The figure shows three views and two pictorial views of one solid part (mm, origin at its lowest corner). Answer the questions. A direction names the side the tool comes from. Give positions to 0.01 mm unless a question says otherwise; leave off trailing zeros. Write each loop counter-clockwise with the first axis right and the second up, starting at its lowest first coordinate (ties: lowest second). Pieces come first, ordered by that corner, then holes. Notation, with made-up numbers: (71, 11) - (106, 11) arc R27 cw to (106, 28) - close; hole circle Ø11 at (-2, 23.5). An arc over 180 degrees is marked (long way). Answer as CSV lines item,"result". Start each with the question number.
(1) Find section B-B (y = 42). Write down the section's boundary in (x, z).
(2) For the marked faces 1 and 2, determine the directions among +Z, -Z, +X, -X, +Y, -Y from which every point of the face is accessible in a straight line to the end or side of a thin tool.
(3) Straight lines are drawn through the part: probe 1 along Y at (x, z) = (13.5, 29.5); probe 2 along Y at (x, z) = (24.35, 25.4) (1 decimal); probe 3 along X at (y, z) = (46.5, 35). For each, find the intervals that lie inside material, in ascending order.
(4) For a pull along X with two mould halves and no side action, classify the marked faces 3, 4, 5 and 6 as pulls with the +X half, pulls with the -X half, needs draft (parallel to the pull), parting line crosses it, or undercut.
(5) Find section C-C (z = 25.4). Write down the section's boundary in (x, y) (1 decimal), then the cut area to 3 significant figures.
(6) Find section A-A (x = 7). Write down the section's boundary in (y, z), then the cut area to 3 significant figures.
(7) Find section D-D (z = 46.5). Write down the section's boundary in (x, y).
(8) Each of these flat-tipped pins is pushed along its axis until it touches: pin 1 Ø4 at (y, z) = (37, 20) entering from +X; pin 2 Ø3.5 at (x, z) = (13.51, 12.7) entering from +Y (3 decimals). Where does it stop, or does it pass through?
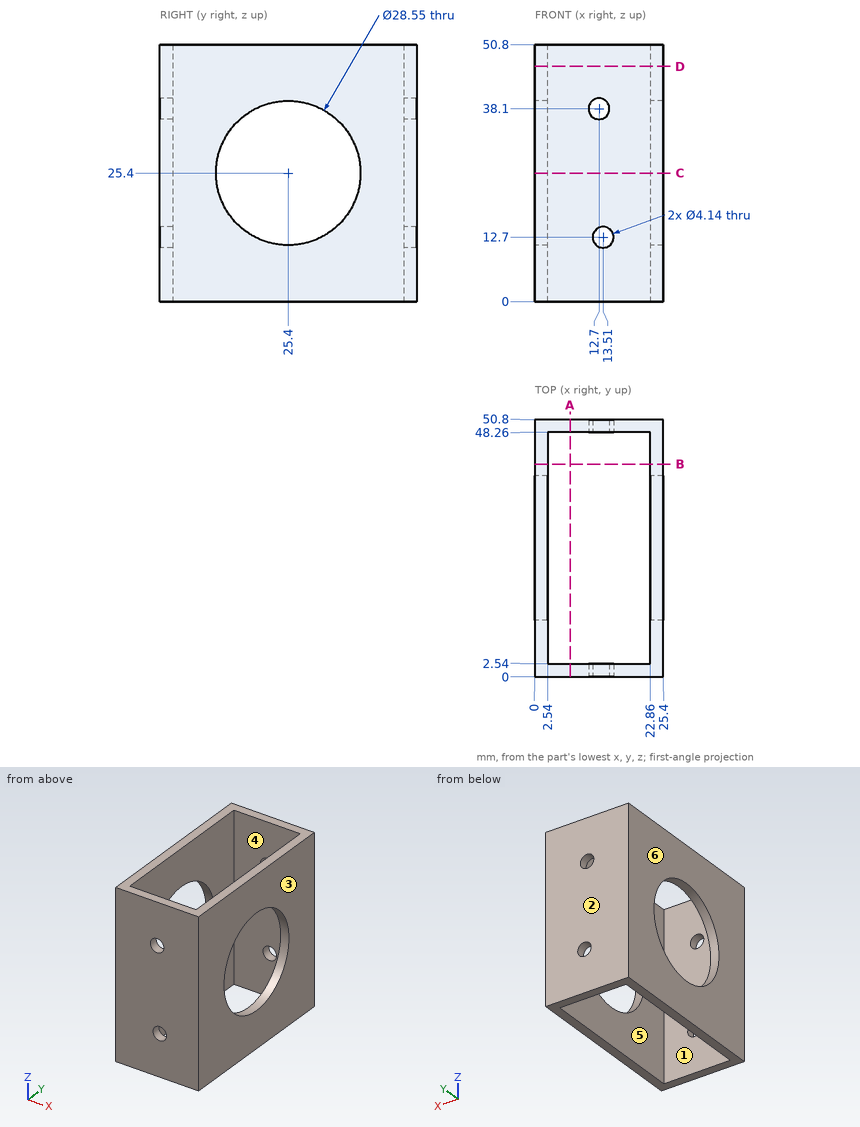
Result set:
1,outline,"(0, 0) - (2.54, 0) - (2.54, 50.8) - (0, 50.8) - close; (22.86, 0) - (25.4, 0) - (25.4, 50.8) - (22.86, 50.8) - close"
2,face 1,"+Z, -Z"
2,face 2,"+Z, -Z, +X, -X, +Y"
3,probe 1,"0 to 2.54, 48.26 to 50.8"
3,probe 2,"0 to 11.1, 39.7 to 50.8"
3,probe 3,"0 to 2.54, 22.86 to 25.4"
4,face 3,"pulls with the +X half"
4,face 4,"undercut"
4,face 5,"undercut"
4,face 6,"pulls with the -X half"
5,outline,"(0, 0) - (25.4, 0) - (25.4, 11.1) - (22.9, 11.1) - (22.9, 2.5) - (2.5, 2.5) - (2.5, 11.1) - (0, 11.1) - close; (0, 39.7) - (2.5, 39.7) - (2.5, 48.3) - (22.9, 48.3) - (22.9, 39.7) - (25.4, 39.7) - (25.4, 50.8) - (0, 50.8) - close"
5,area,"216 mm^2"
6,outline,"(0, 0) - (2.54, 0) - (2.54, 50.8) - (0, 50.8) - close; (48.26, 0) - (50.8, 0) - (50.8, 50.8) - (48.26, 50.8) - close"
6,area,"258 mm^2"
7,outline,"(0, 0) - (25.4, 0) - (25.4, 50.8) - (0, 50.8) - close; hole (2.54, 2.54) - (22.86, 2.54) - (22.86, 48.26) - (2.54, 48.26) - close"
8,pin 1,"x = 25.4"
8,pin 2,"through"
